```python
from build123d import *

# Parameters (mm, degrees)
F1_DEPTH = 50


with BuildPart() as f1:
    # F0 (on Front) → F1 (new body)
    with BuildSketch(Plane.XZ):
        with BuildLine():
            Line((-2.5, 0), (0, 0))
            Line((0, 0), (2.5, 0))
            Line((2.5, 0), (2.5, 2))
            Line((2.5, 2), (2.842854, 2))
            ThreePointArc((2.842854, 2), (2.946854, 2.046917), (2.980508, 2.155933))
            Line((2.980508, 2.155933), (2.51519, 5.878481))
            ThreePointArc((2.51519, 5.878481), (2.469344, 5.965274), (2.377535, 6))
            Line((2.377535, 6), (2.138726, 6))
            ThreePointArc((2.138726, 6), (2.040632, 5.959368), (2, 5.861274))
            Line((2, 5.861274), (2, 1.138726))
            ThreePointArc((2, 1.138726), (1.959368, 1.040632), (1.861274, 1))
            Line((1.861274, 1), (0, 1))
            Line((0, 1), (-1.861274, 1))
            ThreePointArc((-1.861274, 1), (-1.959368, 1.040632), (-2, 1.138726))
            Line((-2, 1.138726), (-2, 5.861274))
            ThreePointArc((-2, 5.861274), (-2.040632, 5.959368), (-2.138726, 6))
            Line((-2.138726, 6), (-2.377535, 6))
            ThreePointArc((-2.377535, 6), (-2.469344, 5.965274), (-2.51519, 5.878481))
            Line((-2.51519, 5.878481), (-2.980508, 2.155933))
            ThreePointArc((-2.980508, 2.155933), (-2.946854, 2.046917), (-2.842854, 2))
            Line((-2.842854, 2), (-2.5, 2))
            Line((-2.5, 2), (-2.5, 0))
        make_face()
    extrude(amount=F1_DEPTH)


solid = f1.part
```
Model file for the job. Use its own axes, mm. A direction names the side the tool comes from. Coordinates: 2 decimals unless noted, no trailing zeros. Loops run counter-clockwise (first coordinate to the right, second up) from the corner with the lowest first, then second, coordinate; pieces in that order, holes last. Notation, with made-up numbers: (16, 11) -> (27, 11) arc R15 cw to (27, 32) -> close; hole circle Ø2 at (37, -30). An arc over 180 degrees is marked (long way). Answer as a JSON object with one key per item and string values.
Q1. Cut at B-B (y = -21.5). List the corners of the cut face in (x, z), and give its area (3 significant figures).
Report:
{"outline": "(-2.98, 2.16) arc R0.14 ccw to (-2.84, 2) -> (-2.5, 2) -> (-2.5, 0) -> (2.5, 0) -> (2.5, 2) -> (2.84, 2) arc R0.14 ccw to (2.98, 2.16) -> (2.52, 5.88) arc R0.14 ccw to (2.38, 6) -> (2.14, 6) arc R0.14 ccw to (2, 5.86) -> (2, 1.14) arc R0.14 cw to (1.86, 1) -> (-1.86, 1) arc R0.14 cw to (-2, 1.14) -> (-2, 5.86) arc R0.14 ccw to (-2.14, 6) -> (-2.38, 6) arc R0.14 ccw to (-2.52, 5.88) -> close", "area": "12.0 mm2"}
Q2. Flat gauge pins, fed straight in: P1, Ø1, axis at y = -13, z = 1, coming from the +X side; P2, Ø1.9, axis at x = 0, y = -28.5, coming from the +Z side. Where does each tip first touch, or does it go through?
Report:
{"P1": "stops at x = 2.5", "P2": "stops at z = 1"}
Q3. Cut at C-C (z = 5.3). List the corners of the cut face in (x, y), and give its area (4 significant figures).
Report:
{"outline": "(-2.59, -50) -> (-2, -50) -> (-2, 0) -> (-2.59, 0) -> close; (2, -50) -> (2.59, -50) -> (2.59, 0) -> (2, 0) -> close", "area": "58.75 mm2"}
Q4. Cut at D-D (x = -0.55). List the corners of the cut face in (y, z), and give its area (3 significant figures).
Report:
{"outline": "(-50, 0) -> (0, 0) -> (0, 1) -> (-50, 1) -> close", "area": "50.0 mm2"}
Q5. 3-axis set-ups, long thin cutter, end or side, ignore diameter. For faces 1 (the flat face through (2.5, -25, 1)), 2 (the flat face through (2, -25, 4)), 3 (the flat face through (-2.745, -24.65, 4.043)): which of +Z, -Z, +X, -X, +Y, -Y reach the whole face in a straight line?
Report:
{"face 1": "-Z, +X, +Y, -Y", "face 2": "+Z, +Y, -Y", "face 3": "+Z, -X, +Y, -Y"}
Q6. Cut at A-A (z = 2.8). List the corners of the cut face in (x, y).
Report:
{"outline": "(-2.9, -50) -> (-2, -50) -> (-2, 0) -> (-2.9, 0) -> close; (2, -50) -> (2.9, -50) -> (2.9, 0) -> (2, 0) -> close"}
Q7. Probe probe 1 along X at (y, z) = (-26.5, 1.3); probe 2 along Z at (x, y) = (1.4, -5); probe 3 along X at (y, z) = (-8, 5.05). List the from-to ranges inside material, lowest first.
Report:
{"probe 1": "x = -2.5 to -2, 2 to 2.5", "probe 2": "z = 0 to 1", "probe 3": "x = -2.62 to -2, 2 to 2.62"}
Q8. Pull direction X, two halves, no side cores. Call faces 4 (the flat face through (-2, -25, 3)), 5 (the flat face through (-2.5, -25, 1)), 6 (the flat face through (-0.9, 0, 0.8)): released by +X, released by -X, zero draft, split by the parting line, or undercut.
Report:
{"face 4": "undercut", "face 5": "released by -X", "face 6": "zero draft"}
